Part model, mm, in its own coordinate system. A direction names the side the tool comes from. Coordinates: 2 decimals unless noted, no trailing zeros. Write each loop counter-clockwise with the first axis right and the second up, starting at its lowest first coordinate (ties: lowest second). Pieces come first, ordered by that corner, then holes. Notation, with made-up numbers: (23.25, 25.5) - (33.25, 25.5) arc R19 cw to (33.25, 58.5) - close; hole circle Ø2 at (-17, 40). An arc over 180 degrees is marked (long way). Use one line per item in the form item = value. Start each with the question number.
from build123d import *

# Parameters (mm, degrees)
SKETCH1_W           = 25.4
SKETCH1_H           = 44.45
BOSS_EXTRUDE1_DEPTH = 12.7
SKETCH2_R           = 2.75
CUT_EXTRUDE1_DEPTH  = 13.7
SKETCH3_R           = 5
CUT_EXTRUDE2_DEPTH  = 9.525
SKETCH5_R           = 0.5953125
CUT_EXTRUDE3_DEPTH  = 13.7
FILLET1_R           = 2.54


with BuildPart() as part:
    # Sketch1 → Boss-Extrude1 (new body)
    with BuildSketch(Plane.XY):
        with Locations((0, 53.975)):
            Rectangle(SKETCH1_W, SKETCH1_H)
    extrude(amount=BOSS_EXTRUDE1_DEPTH)

    # Sketch2 → Cut-Extrude1 (cut, through all)
    with BuildSketch(Plane.XY.offset(12.7)):
        with Locations((0, 50.8)):
            Circle(SKETCH2_R)
        with Locations((0, 69.85)):
            Circle(SKETCH2_R)
    extrude(amount=-CUT_EXTRUDE1_DEPTH, mode=Mode.SUBTRACT)

    # Sketch3 → Cut-Extrude2 (cut)
    with BuildSketch(Plane.XY.offset(12.7)):
        with Locations((0, 50.8)):
            Circle(SKETCH3_R)
        with Locations((0, 69.85)):
            Circle(SKETCH3_R)
    extrude(amount=-CUT_EXTRUDE2_DEPTH, mode=Mode.SUBTRACT)

    # Sketch5 → Cut-Extrude3 (cut, through all)
    with BuildSketch(Plane.XY.offset(12.7)):
        with Locations((7.9375, 41.275)):
            Circle(SKETCH5_R)
        with Locations((-7.9375, 41.275)):
            Circle(SKETCH5_R)
        with Locations((-7.9375, 60.325)):
            Circle(SKETCH5_R)
        with Locations((7.9375, 60.325)):
            Circle(SKETCH5_R)
    extrude(amount=-CUT_EXTRUDE3_DEPTH, mode=Mode.SUBTRACT)

    # Fillet1
    fillet1_edges = [part.edges().sort_by_distance(p)[0] for p in [
        (-12.7, 76.2, 6.35),
        (12.7, 76.2, 6.35),
        (12.7, 31.75, 6.35),
        (-12.7, 31.75, 6.35),
    ]]
    fillet(fillet1_edges, radius=FILLET1_R)


solid = part.part
Q1. Pin check, flat tips, straight feed: P1, Ø9, axis at x = 0, y = 69.85, coming from the +Z side (3 decimals); P2, Ø6, axis at x = -6.5, y = 48, coming from the -Z side. Stop position of each tip, or through.
Q2. Slice it at D-D (y = 50). List the corners of the cut face in (x, z) (3 decimals).
Q3. Slice it at A-A (y = 69.85). List the corners of the cut face in (x, z) (3 decimals).
Q4. Drill centre lines: probe 1 along Y at (x, z) = (8, 6.5); probe 2 along Y at (x, z) = (0, 1.55); probe 3 along X at (y, z) = (72, 11.25). Where is each one in solid material? Low to high.
Q5. Mould opens along Y. For faces 1 (the flat face through (2.2, 67.7, 3.175)), 2 (the flat face through (0, 54, 0)), 3 (the cylindrical face through (11.936, 75.476, 6.439)) say: released by +Y, released by -Y, zero draft, split by the parting line, or undercut.
Q6. Slice it at C-C (z = 6.75). Count the separate pieces of the cut face and the enclosed holes in it, plus the area to 3 significant figures.
Q7. Slice it at B-B (x = 0). List the corners of the cut face in (y, z) (3 decimals).
Q8. Which spindle directions (+Z, -Z, +X, -X, +Y, -Y) get a long thin tool onto all of the face, cutting with end or side? Do faces 4 (the cylindrical face through (-11.976, 32.514, 6.439)), 5 (the flat face through (2.2, 48.6, 3.175)). Say none if no direction does.
Solution:
q1.P1 = 3.175
q1.P2 = 0
q2.outline = (-12.7, 0) - (-2.631, 0) - (-2.631, 3.175) - (-4.936, 3.175) - (-4.936, 12.7) - (-12.7, 12.7) - close; (2.631, 0) - (12.7, 0) - (12.7, 12.7) - (4.936, 12.7) - (4.936, 3.175) - (2.631, 3.175) - close
q3.outline = (-12.7, 0) - (-2.75, 0) - (-2.75, 3.175) - (-5, 3.175) - (-5, 12.7) - (-12.7, 12.7) - close; (2.75, 0) - (12.7, 0) - (12.7, 12.7) - (5, 12.7) - (5, 3.175) - (2.75, 3.175) - close
q4.probe_1 = 31.75 to 40.68, 41.87 to 59.73, 60.92 to 76.2
q4.probe_2 = 31.75 to 48.05, 53.55 to 67.1, 72.6 to 76.2
q4.probe_3 = -12.7 to -4.51, 4.51 to 12.7
q5.face_1 = undercut
q5.face_2 = zero draft
q5.face_3 = released by +Y
q6.separate_pieces = 1
q6.enclosed_holes = 6
q6.area = 962 mm2
q7.outline = (31.75, 0) - (48.05, 0) - (48.05, 3.175) - (45.8, 3.175) - (45.8, 12.7) - (31.75, 12.7) - close; (53.55, 0) - (67.1, 0) - (67.1, 3.175) - (64.85, 3.175) - (64.85, 12.7) - (55.8, 12.7) - (55.8, 3.175) - (53.55, 3.175) - close; (72.6, 0) - (76.2, 0) - (76.2, 12.7) - (74.85, 12.7) - (74.85, 3.175) - (72.6, 3.175) - close
q8.face_4 = +Z, -Z, -X, -Y
q8.face_5 = +Z
